Build history of the part. All positions in model axes, mm. A direction names the side the tool comes from. Round coordinates to 2 decimals unless told otherwise and drop trailing zeros. Write each loop counter-clockwise with the first axis right and the second up, starting at its lowest first coordinate (ties: lowest second). Pieces come first, ordered by that corner, then holes. Notation, with made-up numbers: M 10.25,-34 L 26.25,-34 A14 cw 26.25,-11 Z; hole C 66,-14.75 d2. An arc over 180 degrees is marked long. Write item = value, one per line. Start each with the question number.
Q1. Pull direction Y, two halves, no side cores. Call faces 3 (the flat face through (3, 40.743, 3)), 4 (the cylindrical face through (29.8, -24.57, 3.13)), 5 (the flat face through (35.641, 5, 3)): released by +Y, released by -Y, zero draft, split by the parting line, or undercut.
Q2. Tool access for faces 1 (the flat face through (3, -29.107, 3)), 2 (the flat face through (21, 31.853, 3)): list every direction of +Z, -Z, +X, -X, +Y, -Y with a clear straight run to the whole face (end or side of a thin tool).
Q3. Band-saw the part on D-D on x = -10. Write the cut outline in (y, z).
Q4. Band-saw the part on B-B on x = 29. Write the cut outline in (y, z), plus the area to 3 significant figures.
Q5. Band-saw the part on A-A on y = 13. Write the cut outline in (x, z).
Q6. Probe L1, parallel to Y at x = 22, z = 6; L2, parallel to Y at x = -15, z = 5; L3, parallel to Y at x = -10, z = 5. List the from-to ranges inside material, lowest first.
Q7. Band-saw the part on C-C on y = 5. Write the cut outline in (x, z).
```python
from build123d import *

# Parameters (mm, degrees)
SKETCH1_W           = 63.5
SKETCH1_H           = 69.85
BOSS_EXTRUDE1_DEPTH = 6.35
SKETCH2_R           = 2.54
SKETCH2_W           = 19.05
SKETCH2_H           = 5.08
CUT_EXTRUDE1_DEPTH  = 6.35
FILLET1_R           = 2.54
SKETCH3_W           = 21.59
SKETCH3_H           = 15.875
CUT_EXTRUDE2_DEPTH  = 7.62
FILLET3_R           = 2.54


with BuildPart() as part:
    # Sketch1 → Boss-Extrude1 (new body)
    with BuildSketch(Plane.XY):
        with Locations((3.891179619, 5.817505184)):
            Rectangle(SKETCH1_W, SKETCH1_H)
    extrude(amount=BOSS_EXTRUDE1_DEPTH)

    # Sketch2 → Cut-Extrude1 (cut)
    with BuildSketch(Plane.XY.offset(6.35)):
        with Locations((-21.508820381, 34.392505184)):
            Circle(SKETCH2_R)
        with Locations((3.891179619, 34.392505184)):
            Circle(SKETCH2_R)
        with Locations((-21.508820381, -22.757494816)):
            Circle(SKETCH2_R)
        with Locations((3.891179619, -22.757494816)):
            Circle(SKETCH2_R)
        with Locations((21.036179619, 34.392505184)):
            Rectangle(SKETCH2_W, SKETCH2_H)
        with Locations((21.036179619, -22.757494816)):
            Rectangle(SKETCH2_W, SKETCH2_H)
        with Locations((21.036179619, 5.817505184)):
            Rectangle(SKETCH2_W, SKETCH2_H)
    extrude(amount=-CUT_EXTRUDE1_DEPTH, mode=Mode.SUBTRACT)

    # Fillet1
    fillet1_edges = [part.edges().sort_by_distance(p)[0] for p in [
        (30.561179619, 31.852505184, 3.175),
        (30.561179619, 3.277505184, 3.175),
        (30.561179619, -25.297494816, 3.175),
        (30.561179619, -20.217494816, 3.175),
        (30.561179619, 8.357505184, 3.175),
        (30.561179619, 36.932505184, 3.175),
        (11.511179619, -20.217494816, 3.175),
        (11.511179619, 8.357505184, 3.175),
        (11.511179619, 36.932505184, 3.175),
        (11.511179619, 31.852505184, 3.175),
        (11.511179619, 3.277505184, 3.175),
        (11.511179619, -25.297494816, 3.175),
    ]]
    fillet(fillet1_edges, radius=FILLET1_R - 0.0001)  # a hair under: the kernel refuses the full size

    # Sketch3 → Cut-Extrude2 (cut)
    with BuildSketch(Plane.XY.offset(6.35)):
        Polygon((-17.043797687, -16.407494816), (7.701179619, -16.407494816), (7.701179619, -0.532494816), (7.449059455, -0.532494816), align=None)
        with Locations((21.036179619, -8.469994816)):
            Rectangle(SKETCH3_W, SKETCH3_H)
        Polygon((-24.048820381, -16.407494816), (10.241179619, 5.817505184), (-24.048820381, 28.042505184), align=None)
        Polygon((-17.043797687, 28.042505184), (7.449059455, 12.167505184), (7.701179619, 12.167505184), (7.701179619, 28.042505184), align=None)
        with Locations((21.036179619, 20.105005184)):
            Rectangle(SKETCH3_W, SKETCH3_H)
    extrude(amount=-CUT_EXTRUDE2_DEPTH, mode=Mode.SUBTRACT)

    # Fillet3
    fillet3_edges = [part.edges().sort_by_distance(p)[0] for p in [
        (10.241179619, 5.817505184, 3.175),
    ]]
    fillet(fillet3_edges, radius=FILLET3_R)


solid = part.part
```
Conclusion:
q1.face_3 = released by +Y
q1.face_4 = undercut
q1.face_5 = zero draft
q2.face_1 = +Z, -Z, +X, -X, -Y
q2.face_2 = +Z, -Z
q3.outline = M -29.11,0 L -16.41,0 L -16.41,6.35 L -29.11,6.35 Z; M -11.84,0 L -7.3,0 L -7.3,6.35 L -11.84,6.35 Z; M 18.94,0 L 23.48,0 L 23.48,6.35 L 18.94,6.35 Z; M 28.04,0 L 40.74,0 L 40.74,6.35 L 28.04,6.35 Z
q4.outline = M -29.11,0 L -25.1,0 L -25.1,6.35 L -29.11,6.35 Z; M -20.41,0 L -16.41,0 L -16.41,6.35 L -20.41,6.35 Z; M -0.53,0 L 3.47,0 L 3.47,6.35 L -0.53,6.35 Z; M 8.16,0 L 12.17,0 L 12.17,6.35 L 8.16,6.35 Z; M 28.04,0 L 32.05,0 L 32.05,6.35 L 28.04,6.35 Z; M 36.74,0 L 40.74,0 L 40.74,6.35 L 36.74,6.35 Z
q4.area = 153 mm^2
q5.outline = M -27.86,0 L -24.05,0 L -24.05,6.35 L -27.86,6.35 Z; M -0.84,0 L 6.16,0 L 6.16,6.35 L -0.84,6.35 Z; M 7.7,0 L 10.24,0 L 10.24,6.35 L 7.7,6.35 Z; M 31.83,0 L 35.64,0 L 35.64,6.35 L 31.83,6.35 Z
q6.L1 = -29.11 to -25.3, -20.22 to -16.41, -0.53 to 3.28, 8.36 to 12.17, 28.04 to 31.85, 36.93 to 40.74
q6.L2 = -29.11 to -16.41, -15.08 to -10.54, 22.18 to 26.72, 28.04 to 40.74
q6.L3 = -29.11 to -16.41, -11.84 to -7.3, 18.94 to 23.48, 28.04 to 40.74
q7.outline = M -27.86,0 L -24.05,0 L -24.05,6.35 L -27.86,6.35 Z; M 7.98,0 L 11.65,0 L 11.65,6.35 L 7.98,6.35 Z; M 30.43,0 L 35.64,0 L 35.64,6.35 L 30.43,6.35 Z
